Design review of the part built by this model. Coordinates are the model's own, in mm. A direction names the side the tool comes from. Coordinates: 2 decimals unless noted, no trailing zeros. Loops run counter-clockwise (first coordinate to the right, second up) from the corner with the lowest first, then second, coordinate; pieces in that order, holes last. Notation, with made-up numbers: M -23,14 L 13,14 A36 cw 13,50 Z; hole C -10.5,0.5 d9. An arc over 180 degrees is marked long. Answer as a JSON object with one key per item and string values. Group by question number.
1. Draft analysis for pull direction Z (two halves, no side actions). For faces 1 (the flat face through (-7, -1.5, 5)), 2 (the flat face through (0, 0.3, 25)), 3 (the flat face through (0, -2, 0)), state which applies: +Z half, -Z half, draft (parallel to the pull), parting line (faces both ways), or undercut.
2. Machinability: for faces 4 (the flat face through (-5, 0.3, 25)), 5 (the flat face through (-0.11, 0.53, 0.38)), 6 (the cylindrical face through (5.8, 0.5, 5.5)), 7 (the flat face through (0, 2.5, 10)), 8 (the cylindrical face through (-0.456, 2.254, 16.655)), which of the approach directions +Z, -Z, +X, -X, +Y, -Y give a long, thin tool a straight path to every point of the face, cutting with its end or side? Answer none if there is none.
3. Insertion check: pin 1 (1.8 mm diameter, centred on x = 4.5, z = 26.5, fed in from +Y); pin 2 (0.7 mm diameter, centred on y = 0, z = 28, fed in from +X); pin 3 (2 mm diameter, centred on x = -7, z = 5, fed in from +Y). Each pin has a flat end and moves straight along its axis. Give the tip position at first contact, or say it passes through.
4. To check wall thickness, follow probe 1 along X at (y, z) = (0.25, 21); probe 2 along X at (y, z) = (0.7, 5.5); probe 3 along X at (y, z) = (2.3, 3) (1 decimal). State the ranges of each line that lie inside material, in increasing order.
5. Consider section A-A (z = 5.5). State the section outline as (x, y) points, then the cut area to 3 significant figures.
6. Consider section C-C (y = -1.1). State the section outline as (x, z) points (3 decimals).
from build123d import *
from OCP.BRepFilletAPI import BRepFilletAPI_MakeChamfer

# Parameters (mm, degrees)
SKETCH1_W                = 15.6
SKETCH1_H                = 5
BOSS_EXTRUDE1_DEPTH      = 20
CHAMFER1_SIZE            = 4
CHAMFER1_SIZE2           = 0.75
SKETCH2_R                = 1.8
CUT_EXTRUDE1_DEPTH       = 23.041778513
SKETCH3_R                = 2
CUT_EXTRUDE2_DEPTH       = 4
SKETCH4_R                = 0.625
CUT_EXTRUDE3_DEPTH       = 0.5
SKETCH5_R                = 0.75
CUT_EXTRUDE4_DEPTH       = 0.5
BOSS_EXTRUDE2_DEPTH      = 0.3
BOSS_EXTRUDE2_DEPTH_BACK = 0.3


with BuildPart() as part:
    # Sketch1 → Boss-Extrude1 (new body)
    with BuildSketch(Plane.XY):
        Rectangle(SKETCH1_W, SKETCH1_H)
    extrude(amount=BOSS_EXTRUDE1_DEPTH)

    # Chamfer1: one chamfer whose edges measure the first distance from different faces: ONE call of the kernel's chamfer builder (chamfer() names one face for all edges)
    chamfer1_edges_1 = [part.edges().sort_by_distance(p)[0] for p in [
        (0, 2.5, 20),
    ]]
    chamfer1_side_1 = [part.faces().sort_by_distance(p)[0] for p in [
        (0, 0, 20),
    ]]
    chamfer1_edges_2 = [part.edges().sort_by_distance(p)[0] for p in [
        (0, 2.5, 0),
    ]]
    chamfer1_side_2 = [part.faces().sort_by_distance(p)[0] for p in [
        (0, 0, 0),
    ]]
    chamfer1_edges_3 = [part.edges().sort_by_distance(p)[0] for p in [
        (-7.8, 2.5, 10),
    ]]
    chamfer1_side_3 = [part.faces().sort_by_distance(p)[0] for p in [
        (-7.8, 0, 10),
    ]]
    chamfer1_edges_4 = [part.edges().sort_by_distance(p)[0] for p in [
        (7.8, 2.5, 10),
    ]]
    chamfer1_side_4 = [part.faces().sort_by_distance(p)[0] for p in [
        (7.8, 0, 10),
    ]]
    chamfer1 = BRepFilletAPI_MakeChamfer(part.part.solid().wrapped)
    for e in chamfer1_edges_1:
        chamfer1.Add(CHAMFER1_SIZE, CHAMFER1_SIZE2, e.wrapped, chamfer1_side_1[0].wrapped)  # the first distance lies on this face
    for e in chamfer1_edges_2:
        chamfer1.Add(CHAMFER1_SIZE, CHAMFER1_SIZE2, e.wrapped, chamfer1_side_2[0].wrapped)  # the first distance lies on this face
    for e in chamfer1_edges_3:
        chamfer1.Add(CHAMFER1_SIZE, CHAMFER1_SIZE2, e.wrapped, chamfer1_side_3[0].wrapped)  # the first distance lies on this face
    for e in chamfer1_edges_4:
        chamfer1.Add(CHAMFER1_SIZE, CHAMFER1_SIZE2, e.wrapped, chamfer1_side_4[0].wrapped)  # the first distance lies on this face
    add(Compound.cast(chamfer1.Shape()), mode=Mode.REPLACE)

    # Sketch2 → Cut-Extrude1 (cut, through all)
    with BuildSketch(Plane(origin=(0, 2.5, 0), x_dir=(1, 0, 0), z_dir=(0, 1, 0))):
        with Locations(Location((0, -5.5, 0), (0, 0, 270))):
            Circle(SKETCH2_R)
    extrude(amount=-CUT_EXTRUDE1_DEPTH, mode=Mode.SUBTRACT)

    # Sketch3 → Cut-Extrude2 (cut)
    with BuildSketch(Plane(origin=(0, 2.5, 0), x_dir=(1, 0, 0), z_dir=(0, 1, 0))):
        with Locations((-7.8, -5.5)):
            Circle(SKETCH3_R)
        with Locations((7.8, -5.5)):
            Circle(SKETCH3_R)
    extrude(amount=-CUT_EXTRUDE2_DEPTH, mode=Mode.SUBTRACT)

    # Sketch4 → Cut-Extrude3 (cut)
    with BuildSketch(Plane(origin=(0, 2.5, 0), x_dir=(1, 0, 0), z_dir=(0, 1, 0))):
        with Locations(Location((4.25, -3, 0), (0, 0, 270))):
            Circle(SKETCH4_R)
        with Locations(Location((-4.25, -3, 0), (0, 0, 90))):
            Circle(SKETCH4_R)
    extrude(amount=-CUT_EXTRUDE3_DEPTH, mode=Mode.SUBTRACT)

    # Sketch5 → Cut-Extrude4 (cut)
    with BuildSketch(Plane(origin=(0, 2.5, 0), x_dir=(1, 0, 0), z_dir=(0, 1, 0))):
        with Locations(Location((0, -17.25, 0), (0, 0, 270))):
            Circle(SKETCH5_R)
    extrude(amount=-CUT_EXTRUDE4_DEPTH, mode=Mode.SUBTRACT)

    # Sketch6 → Boss-Extrude2 (add, two sides: drawn at the far end of the back side and taken through both)
    with BuildSketch(Plane(origin=(0, 0, 0), x_dir=(-1, 0, 0), z_dir=(0, -1, 0)).offset(-BOSS_EXTRUDE2_DEPTH_BACK)):
        Polygon((6.05, -24), (4.85, -24), (4.85, -33.6), (5.25, -34.2), (5.65, -34.2), (6.05, -33.6), align=None)
        Polygon((6.05, -19.25), (3.85, -19.25), (3.85, -20), (3.85, -24), (4.85, -24), (6.05, -24), (6.05, -20), align=None)
        Polygon((-1.6, -19.25), (-1.6, -24), (-0.6, -24), (0, -24), (0.6, -24), (1.6, -24), (1.6, -19.25), align=None)
        Polygon((-6.05, -20), (-6.05, -24), (-4.85, -24), (-3.85, -24), (-3.85, -20), (-3.85, -19.25), (-6.05, -19.25), align=None)
        Polygon((0.6, -24), (0, -24), (0, -34.2), (0.2, -34.2), (0.6, -33.6), align=None)
        Polygon((0, -24), (-0.6, -24), (-0.6, -33.6), (-0.2, -34.2), (0, -34.2), align=None)
        Polygon((-4.85, -24), (-6.05, -24), (-6.05, -33.6), (-5.65, -34.2), (-5.25, -34.2), (-4.85, -33.6), align=None)
    extrude(amount=BOSS_EXTRUDE2_DEPTH + BOSS_EXTRUDE2_DEPTH_BACK)


solid = part.part
Findings below:
{
 "1": {"face 1": "undercut", "face 2": "draft", "face 3": "-Z half"},
 "2": {"face 4": "+Z, +X, -X, +Y", "face 5": "-Z, +X, -X, +Y", "face 6": "+X, +Y", "face 7": "+Z, -Z, +X, -X, +Y", "face 8": "+Y"},
 "3": {"pin 1": "stops at y = 0.3", "pin 2": "stops at x = 6.05", "pin 3": "stops at y = -1.5"},
 "4": {"probe 1": "x = -6.05 to -3.85, -1.6 to 1.6, 3.85 to 6.05", "probe 2": "x = -5.8 to -1.8, 1.8 to 5.8", "probe 3": "x = -7.1 to -4.9, -3.6 to 3.6, 4.9 to 7.1"},
 "5": {"outline": "M -7.8,-2.5 L -1.8,-2.5 L -1.8,2.5 L -5.8,2.5 L -5.8,-1.5 L -7.8,-1.5 Z; M 1.8,-2.5 L 7.8,-2.5 L 7.8,-1.5 L 5.8,-1.5 L 5.8,2.5 L 1.8,2.5 Z", "area": "44.0 mm^2"},
 "6": {"outline": "M -7.725,0.075 L 7.725,0.075 L 7.725,3.501 A2 cw 7.725,7.499 L 7.725,19.925 L -7.725,19.925 L -7.725,7.499 A2 cw -7.725,3.501 Z; hole C 0,5.5 d3.6"}
}
